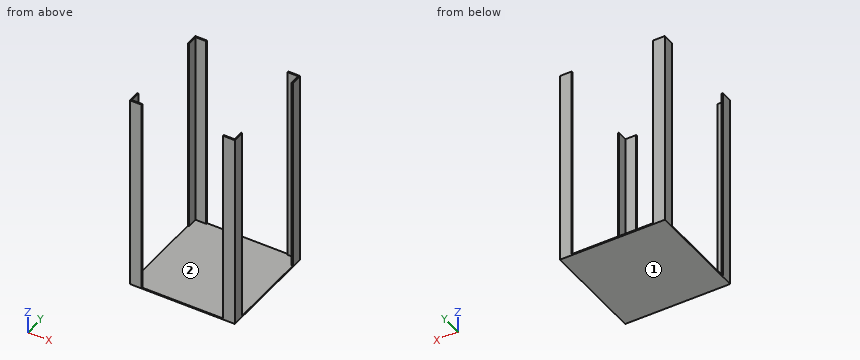
```python
from build123d import *

# Parameters (mm, degrees)
F1_DEPTH = 1000
F2_DEPTH = 6


with BuildPart() as f1:
    # F0 (on Top) → F1 (new body)
    with BuildSketch(Plane.XY):
        Polygon((0, 535), (0, 475), (6, 475), (6, 529), (60, 529), (60, 535), align=None)
    extrude(amount=F1_DEPTH)



with BuildPart() as f1b:
    # F0 (on Top) → F1, piece 2 (new body)
    with BuildSketch(Plane.XY):
        Polygon((529, 475), (535, 475), (535, 535), (475, 535), (475, 529), (529, 529), align=None)
    extrude(amount=F1_DEPTH)


with BuildPart() as f1c:
    # F0 (on Top) → F1, piece 3 (new body)
    with BuildSketch(Plane.XY):
        Polygon((475, 6), (475, 0), (535, 0), (535, 60), (529, 60), (529, 6), align=None)
    extrude(amount=F1_DEPTH)


with BuildPart() as f1d:
    # F0 (on Top) → F1, piece 4 (new body)
    with BuildSketch(Plane.XY):
        Polygon((0, 60), (0, 0), (60, 0), (60, 6), (6, 6), (6, 60), align=None)
    extrude(amount=F1_DEPTH)


with BuildPart() as f1_1:
    add(f1.part)

    add(f1b.part)  # F2 merges F1b

    add(f1c.part)  # F2 merges F1c

    add(f1d.part)  # F2 merges F1d
    # F0 (on Top) → F2 (join)
    with BuildSketch(Plane.XY):
        Polygon((0, 60), (0, 0), (60, 0), (60, 6), (6, 6), (6, 60), align=None)
        Polygon((60, 6), (60, 0), (475, 0), (475, 6), (529, 6), (529, 60), (535, 60), (535, 475), (529, 475), (529, 529), (475, 529), (475, 535), (60, 535), (60, 529), (6, 529), (6, 475), (0, 475), (0, 60), (6, 60), (6, 6), align=None)
        Polygon((475, 6), (475, 0), (535, 0), (535, 60), (529, 60), (529, 6), align=None)
        Polygon((0, 535), (0, 475), (6, 475), (6, 529), (60, 529), (60, 535), align=None)
        Polygon((529, 475), (535, 475), (535, 535), (475, 535), (475, 529), (529, 529), align=None)
    extrude(amount=-F2_DEPTH)


solid = f1_1.part
```
The listing builds one solid part. Answer for the finished solid, in the listing's coordinates (mm). Face numbers are marked on the shaded views. Coordinates: 2 decimals unless noted, no trailing zeros. Write each loop counter-clockwise with the first axis right and the second up, starting at its lowest first coordinate (ties: lowest second). Pieces come first, ordered by that corner, then holes. Notation, with made-up numbers: (-28, -19) -> (-13, -19) arc R32 cw to (-13, 20) -> close; hole circle Ø2 at (-36, -16). An arc over 180 degrees is marked (long way). Write each question's results on one line, items separated by ' | '. Start each with the question number.
1) Flat-ended cylindrical pins translate along their axes: pin 1 Ø1.8 at (y, z) = (3, 540.5) entering from -X; pin 2 Ø1 at (x, y) = (369, 115.5) entering from +Z; pin 3 Ø8 at (x, z) = (468.5, 645) entering from -Y. Find the tip coordinate at first contact, or state that the pin passes through.
2) A cutting plane is placed at A-A (z = 878). Determine the outline of the cut face in (x, y), then the cut area to 3 significant figures.
3) A cutting plane is placed at B-B (y = 251). Determine the outline of the cut face in (x, z).
4) Straight lines are drawn through the part: probe 1 along X at (y, z) = (499, 863.5); probe 2 along Z at (x, y) = (449, 329). For each, find the intervals that lie inside material, in ascending order.
5) For a pull along X with two mould halves and no side action, classify the marked faces 1 and 2 as +X half, -X half, draft (parallel to the pull), parting line (faces both ways), or undercut.
Values follow:
1) pin 1: x = 0 | pin 2: z = 0 | pin 3: through
2) outline: (0, 0) -> (60, 0) -> (60, 6) -> (6, 6) -> (6, 60) -> (0, 60) -> close; (0, 475) -> (6, 475) -> (6, 529) -> (60, 529) -> (60, 535) -> (0, 535) -> close; (475, 0) -> (535, 0) -> (535, 60) -> (529, 60) -> (529, 6) -> (475, 6) -> close; (475, 529) -> (529, 529) -> (529, 475) -> (535, 475) -> (535, 535) -> (475, 535) -> close | area: 2,740 mm²
3) outline: (0, -6) -> (535, -6) -> (535, 0) -> (0, 0) -> close
4) probe 1: 0 to 6, 529 to 535 | probe 2: -6 to 0
5) face 1: draft | face 2: undercut
